Part model, mm, in its own coordinate system. A direction names the side the tool comes from. Round coordinates to 2 decimals unless told otherwise and drop trailing zeros. Return JSON: item names as keys, results as strings. Group by question number.
(1) Drop flat-ended pins along their axis: pin 1 Ø4.5 at (x, z) = (290.5, 78.5) entering from -Y; pin 2 Ø10 at (x, y) = (164.5, -21.5) entering from -Z; pin 3 Ø1.5 at (x, z) = (164.5, 90.5) entering from +Y. Give the stop position or say it passes through.
(2) Drill centre lines: L1, parallel to Y at x = 194, z = 46; L2, parallel to Y at x = 192, z = 72.5; L3, parallel to X at y = -50.5, z = 115. Where is each one in solid material? Low to high. Write a range as from..to.
(3) Mould opens along Z. For faces 6 (the flat face through (271.2, -67.853, 126.4)), 7 (the flat face through (149.93, -19.56, 81.25)), 8 (the flat face through (270.884, -71.915, 126.582)) say: +Z half, -Z half, draft (parallel to the pull), parting line (faces both ways), or undercut.
(4) Tool access for faces 1 (the flat face through (129.616, -9.809, 74.834)), 2 (the cylindrical face through (291.5, -70.4, 77)), 3 (the flat face through (289.1, -67.853, 77.3)), 4 (the cylindrical face through (255.42, -50.09, 3.08)), 5 (the flat face through (288.75, -71.92, 77.62)): list every direction of +Z, -Z, +X, -X, +Y, -Y with a clear straight run to the whole face (end or side of a thin tool).
from build123d import *

# Parameters (mm, degrees)
REVOLVE1_ANGLE      = 30
SKETCH8_R           = 20
CUT_EXTRUDE1_DEPTH  = 10
SKETCH9_R           = 1.65
BOSS_EXTRUDE1_DEPTH = 3
BOSS_EXTRUDE2_DEPTH = 7.5
SKETCH10_R          = 2.75
CUT_EXTRUDE2_DEPTH  = 322.291633421
CIRPATTERN1_COUNT   = 3
CIRPATTERN1_ANGLE   = 20


with BuildPart() as part:
    # Sketch7 → Revolve1 (revolve)
    with BuildSketch(Plane.XY):
        with BuildLine():
            Line((45, 1.5), (0, 1.5))
            Line((0, 1.5), (0, -0.5))
            Line((0, -0.5), (0.5, -0.5))
            Line((0.5, -0.5), (45, -0.5))
            ThreePointArc((45, -0.5), (176.353256324, -17.04581533), (299.5, -65.649534053))
            Line((299.5, -65.649534053), (299.5, -85.057353814))
            Line((299.5, -85.057353814), (299.5, -87.3365737))
            ThreePointArc((299.5, -87.3365737), (300.500587667, -86.78965163), (301.5, -86.24058477))
            Line((301.5, -86.24058477), (301.5, -64.466303097))
            ThreePointArc((301.5, -64.466303097), (177.423377038, -15.255605667), (45, 1.5))
        make_face()
    revolve(axis=Axis((0, 0, 0), (0, -1, 0)), revolution_arc=REVOLVE1_ANGLE)

    # Sketch8 → Cut-Extrude1 (cut)
    with BuildSketch(Plane(origin=(0, 1.5, 0), x_dir=(1, 0, 0), z_dir=(0, 1, 0))):
        Circle(SKETCH8_R)
    extrude(amount=-CUT_EXTRUDE1_DEPTH, mode=Mode.SUBTRACT)

    # Sketch9 → Boss-Extrude1 (add)
    with BuildSketch(Plane(origin=(0, 0, 1.6), x_dir=(-1, 0, 0), z_dir=(0, 0, -1))):
        with BuildLine():
            ThreePointArc((-47.477373191, -0.005788221), (-173.847460419, -15.895397549), (-292.781250831, -61.465476862))
            Line((-292.781250831, -61.465476862), (-279.669089435, -61.465476862))
            ThreePointArc((-279.669089435, -61.465476862), (-255.073001384, -49.937778659), (-229.91274685, -39.699762977))
            ThreePointArc((-229.91274685, -39.699762977), (-227.597805944, -39.782747629), (-226.032061896, -41.489874873))
            Line((-226.032061896, -41.489874873), (-223.847573085, -47.552153691))
            ThreePointArc((-223.847573085, -47.552153691), (-220.219756041, -50.565420802), (-215.82374839, -48.857804945))
            Line((-215.82374839, -48.857804945), (-214.925668504, -46.947888182))
            Line((-214.925668504, -46.947888182), (-208.423927791, -33.120851453))
            ThreePointArc((-208.423927791, -33.120851453), (-207.69256892, -32.146690461), (-206.634183209, -31.543619054))
            ThreePointArc((-206.634183209, -31.543619054), (-144.562309401, -15.54254357), (-81.001445464, -7.237815383))
            Line((-81.001445464, -7.237815383), (-75.885042341, -16.035876247))
            ThreePointArc((-75.885042341, -16.035876247), (-72.834885241, -18.246061874), (-69.148521267, -17.472046696))
            Line((-69.148521267, -17.472046696), (-68.664438088, -17.071211426))
            Line((-68.664438088, -17.071211426), (-55.418958748, -6.103560573))
            Line((-55.418958748, -6.103560573), (-47.477373191, -0.005788221))
        make_face()
        with Locations((-219.472922513, -45.975786864)):
            Circle(SKETCH9_R, mode=Mode.SUBTRACT)
        with Locations((-71.865332392, -13.698263805)):
            Circle(SKETCH9_R, mode=Mode.SUBTRACT)
    boss_extrude1 = extrude(amount=-BOSS_EXTRUDE1_DEPTH)

    # Mirror1: Boss-Extrude1 across plane
    add(boss_extrude1.mirror(Plane(origin=(0, 0, 0), x_dir=(0.9659258262890681, 0, 0.2588190451025213), z_dir=(0.2588190451025213, 0, -0.9659258262890682))))

    # Sketch11 → Boss-Extrude2 (add, symmetric)
    with BuildSketch(Plane(origin=(0, -75.353443934, 0), x_dir=(1, 0, 0), z_dir=(0, 1, 0))):
        with BuildLine():
            Line((296.354521141, -43.29258365), (299.369908318, -8.826550513))
            ThreePointArc((299.369908318, -8.826550513), (298.360312078, -26.103144953), (296.354521141, -43.29258365))
        make_face()
    boss_extrude2 = extrude(amount=BOSS_EXTRUDE2_DEPTH, both=True)

    # Sketch10 → Cut-Extrude2 (cut, through all)
    with BuildSketch(Plane(origin=(300.352701475, 0, 26.277456438), x_dir=(0.08715574274765836, 0, -0.9961946980917455), z_dir=(0.9961946980917457, 0, 0.08715574274765837))):
        with Locations((0, -75.353443934)):
            Circle(SKETCH10_R)
    cut_extrude2 = extrude(amount=-CUT_EXTRUDE2_DEPTH, mode=Mode.SUBTRACT)

    # CirPattern1: Boss-Extrude2, Cut-Extrude2 ×3 about axis
    cirpattern1_axis = Axis((0, 0, 0), (0, -1, 0))
    add([boss_extrude2.rotate(cirpattern1_axis, i * CIRPATTERN1_ANGLE / (CIRPATTERN1_COUNT - 1)) for i in range(1, CIRPATTERN1_COUNT)])
    add([cut_extrude2.rotate(cirpattern1_axis, i * CIRPATTERN1_ANGLE / (CIRPATTERN1_COUNT - 1)) for i in range(1, CIRPATTERN1_COUNT)], mode=Mode.SUBTRACT)


solid = part.part
Computed values:
{
 "1": {"pin 1": "y = -87.34", "pin 2": "z = 1.6", "pin 3": "y = -17.81"},
 "2": {"L1": "-23.5..-21.41", "L2": "-25.32..-23.22", "L3": "243.89..249.05"},
 "3": {"face 6": "draft", "face 7": "undercut", "face 8": "-Z half"},
 "4": {"face 1": "+Z, -X, +Y, -Y", "face 2": "+Z, +X, +Y, -Y", "face 3": "-Z, -X", "face 4": "-Z, -Y", "face 5": "-Z, -X, -Y"}
}
